Source: CAD feature listing. Evaluate the final solid. Frame: model axes, mm. A direction names the side the tool comes from. Coordinates: 2 decimals unless noted, no trailing zeros. Order: outer loops, then holes, each group sorted by start corner. A loop starts at its lowest first (then second) coordinate and runs counter-clockwise, first axis right, second up.
Item 1: Mould query, pull axis X, two halves, no side actions, for faces 1 (the conical face through (27.372, 8.117, -12.497)), 2 (the cylindrical face through (-29.226, -0.175, -0.57)), 3 (the flat face through (0, 12.5, -4)). Classes: released by +X, released by -X, zero draft, split by the parting line, or undercut.
Item 2: Ray query, line 1 (Y direction, x = 27.5, z = -5); line 2 (X direction, y = -8, z = -7); line 3 (X direction, y = 8, z = -3). Return the intervals inside material, ascending.
Item 3: Contact query for a flat-ended pin moving along its axis: P1, Ø7.5, axis at x = 12.5, y = 6, coming from the -Z side. Output: stop coordinate, or through.
Item 4: Section A-A on z = -6. Return the cut outline in (x, y).
Item 5: Section C-C on z = -15.5. Return the cut outline in (x, y), then the cut area to 3 significant figures.
Item 6: Reachability of faces 4 (the cylindrical face through (27.63, -7.01, -6.08)), 5 (the flat face through (2, 0, 0)), 6 (the flat face through (0, 0, -5)) from +Z, -Z, +X, -X, +Y, -Y: full face, straight path, thin tool, end or side. Return the list, or none.
Item 7: Section B-B on y = -2.25. Return the cut outline in (x, z).
Item 8: Section D-D on x = -19. Return the cut outline in (y, z).
from build123d import *

# Parameters (mm, degrees)
F1_DEPTH = 12.5
F3_R     = 2
F4_D     = 2
F4_DEPTH = 12
F4_TIP   = 0.600860619


# Not quite as in the source:
# - a feature names something its author has since deleted; it is built from what else it names


with BuildPart() as f1:
    # F0 (on Front) → F1 (new body, symmetric)
    with BuildSketch(Plane.XZ):
        Polygon((30.1726347237, 0), (-29.8273652763, 0), (-29.8273652763, -25), (-24.8273652763, -25), (-24.8273652763, -5), (25.1726347237, -5), (25.1726347237, -25), (30.1726347237, -25), align=None)
    extrude(amount=F1_DEPTH, both=True)

    # F3
    f3_edges = [f1.edges().sort_by_distance(p)[0] for p in [
        (30.172635, 0, -25),
        (-29.827365, 0, -25),
        (-29.827365, 0, 0),
    ]]
    fillet(f3_edges, radius=F3_R)

    # F4
    with Locations(Plane.XY):
        with Locations((27.5, 8), (27.5, -8)):
            Hole(F4_D / 2, depth=F4_DEPTH)
            with Locations((0, 0, -(F4_DEPTH + F4_TIP / 2))):  # 118° drill point
                Cone(0, F4_D / 2, F4_TIP, mode=Mode.SUBTRACT)


solid = f1.part
Answer list:
1. face 1: undercut
1. face 2: released by -X
1. face 3: zero draft
2. line 1: y = -12.5 to -9, -7 to 7, 9 to 12.5
2. line 2: x = -29.83 to -24.83, 25.17 to 26.5, 28.5 to 30.17
2. line 3: x = -29.83 to 26.5, 28.5 to 30.17
3. P1: stops at z = -5
4. outline: (-29.83, -12.5) - (-24.83, -12.5) - (-24.83, 12.5) - (-29.83, 12.5) - close; (25.17, -12.5) - (30.17, -12.5) - (30.17, 12.5) - (25.17, 12.5) - close; hole circle Ø2 at (27.5, -8); hole circle Ø2 at (27.5, 8)
5. outline: (-29.83, -12.5) - (-24.83, -12.5) - (-24.83, 12.5) - (-29.83, 12.5) - close; (25.17, -12.5) - (30.17, -12.5) - (30.17, 12.5) - (25.17, 12.5) - close
5. area: 250 mm2
6. face 4: +Z
6. face 5: +Z, +X, -X, +Y, -Y
6. face 6: -Z, +Y, -Y
7. outline: (-29.83, -23) arc R2 ccw to (-27.83, -25) - (-24.83, -25) - (-24.83, -5) - (25.17, -5) - (25.17, -25) - (28.17, -25) arc R2 ccw to (30.17, -23) - (30.17, 0) - (-27.83, 0) arc R2 ccw to (-29.83, -2) - close
8. outline: (-12.5, -5) - (12.5, -5) - (12.5, 0) - (-12.5, 0) - close
